Check sheet for the drawn part. Datum: minimum x, y, z corner. Units: mm. A direction names the side the tool comes from. Give positions to 0.01 mm unless a question says otherwise; leave off trailing zeros. Loops run counter-clockwise (first coordinate to the right, second up) from the corner with the lowest first, then second, coordinate; pieces in that order, holes last. Notation, with made-up numbers: (83, -31.5) - (117, -31.5) arc R18 ccw to (117, 3.5) - close; hole circle Ø8 at (61, -26). An arc over 180 degrees is marked (long way). Answer in a Markdown table with one row per item.
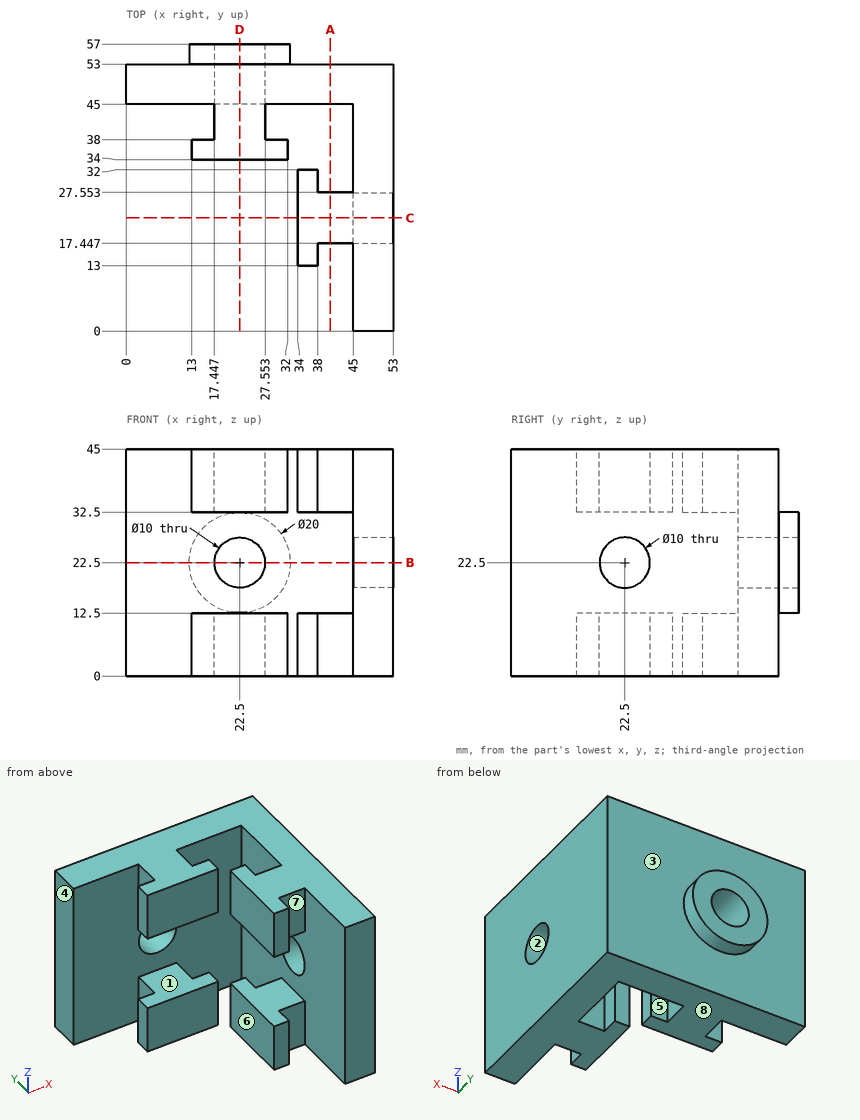
Q1. Sectioned sample at D-D (x = 22.5). Record the cut outline in (y, z).
Completed:
| item | result |
|---|---|
| outline | (34, 0) - (53, 0) - (53, 12.5) - (57, 12.5) - (57, 17.5) - (45, 17.5) - (45, 12.5) - (34, 12.5) - close; (34, 32.5) - (45, 32.5) - (45, 27.5) - (57, 27.5) - (57, 32.5) - (53, 32.5) - (53, 45) - (34, 45) - close |
Q2. Draft check along Y on the marked faces 1, 2 and 3. Enter one of: +Y half, -Y half, draft (parallel to the pull), parting line (faces both ways), or undercut.
Completed:
| item | result |
|---|---|
| face 1 | draft |
| face 2 | undercut |
| face 3 | +Y half |
Q3. Sectioned sample at A-A (x = 40.5). Record the cut outline in (y, z).
Completed:
| item | result |
|---|---|
| outline | (17.45, 0) - (27.55, 0) - (27.55, 12.5) - (17.45, 12.5) - close; (17.45, 32.5) - (27.55, 32.5) - (27.55, 45) - (17.45, 45) - close; (45, 0) - (53, 0) - (53, 45) - (45, 45) - close |
Q4. Thickness scan on line 1 (Z direction, x = 22.5, y = 49); line 2 (Z direction, x = 22.5, y = 54.5); line 3 (Y direction, x = 49, z = 22.5). Record the ranges inside material, lowest first.
Completed:
| item | result |
|---|---|
| line 1 | 0 to 17.5, 27.5 to 45 |
| line 2 | 12.5 to 17.5, 27.5 to 32.5 |
| line 3 | 0 to 17.5, 27.5 to 53 |
Q5. Sectioned sample at C-C (y = 22.5). Record the cut outline in (x, z), and give its area (3 significant figures).
Completed:
| item | result |
|---|---|
| outline | (34, 0) - (53, 0) - (53, 17.5) - (45, 17.5) - (45, 12.5) - (34, 12.5) - close; (34, 32.5) - (45, 32.5) - (45, 27.5) - (53, 27.5) - (53, 45) - (34, 45) - close |
| area | 555 mm^2 |
Q6. Go/stop test with flat-tipped pins: P1, Ø2, axis at x = 29.5, z = 37.5, coming from the +Y side; P2, Ø5, axis at y = 38, z = 39, coming from the -X side; P3, Ø3, axis at y = 15, z = 15.5, coming from the -X side. Record where each tip stops, or that it passes through.
Completed:
| item | result |
|---|---|
| P1 | y = 53 |
| P2 | x = 13 |
| P3 | x = 45 |
Q7. Sectioned sample at B-B (z = 22.5). Record the cut outline in (x, y).
Completed:
| item | result |
|---|---|
| outline | (0, 45) - (17.5, 45) - (17.5, 57) - (12.5, 57) - (12.5, 53) - (0, 53) - close; (27.5, 45) - (45, 45) - (45, 27.5) - (53, 27.5) - (53, 53) - (32.5, 53) - (32.5, 57) - (27.5, 57) - close; (45, 0) - (53, 0) - (53, 17.5) - (45, 17.5) - close |
Q8. Tool access check on the marked faces 4, 5, 6, 7 and 8. Record the directions out of +Z, -Z, +X, -X, +Y, -Y that give a thin tool (end or side, any length) a straight path to the whole face; none if there is none.
Completed:
| item | result |
|---|---|
| face 4 | +Z, -Z, -X, +Y, -Y |
| face 5 | +Z, -Z |
| face 6 | +Z, -Z, -X, -Y |
| face 7 | +Z, -Z, -Y |
| face 8 | -Z, +X, -X, +Y, -Y |
